Verification items for this drawing (mm, ordinates from the low corner). Give positions to 0.01 mm unless a question says otherwise; leave off trailing zeros. Write each loop counter-clockwise with the first axis right and the second up, starting at its lowest first coordinate (ties: lowest second). Pieces come first, ordered by that corner, then holes. Notation, with made-up numbers: M 71.25,-3.5 L 79.25,-3.5 A21 cw 79.25,30.5 Z; hole C -21,-19 d11. An arc over 180 degrees is marked long. Use one line per item in the form item = value. Start each with the question number.
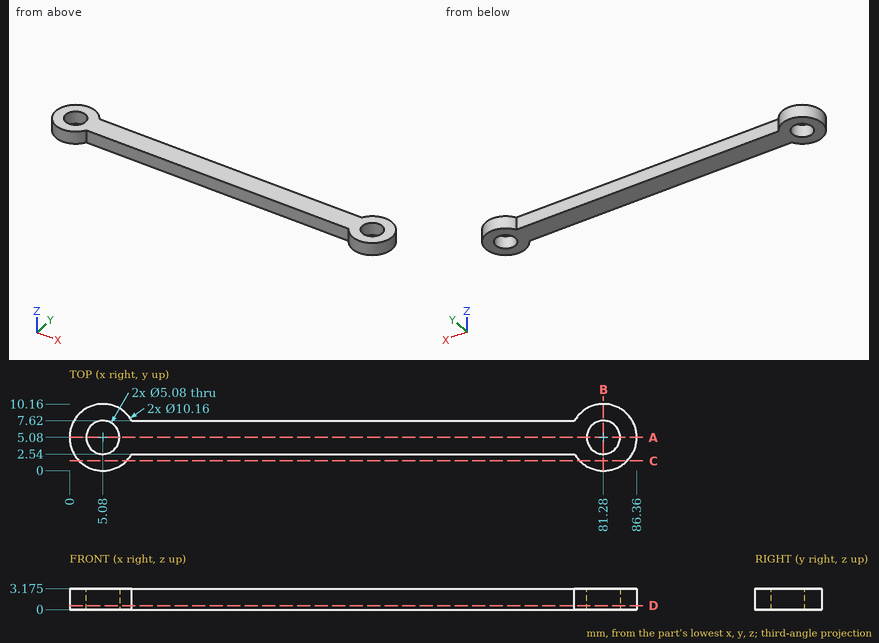
(1) Sectioned sample at C-C, the plane y = 1.5. Record the boundary of the cut face in (x, z) (3 decimals), plus the area to 3 significant figures.
(2) Sectioned sample at B-B, the plane x = 81.28. Record the boundary of the cut face in (y, z) (3 decimals).
(3) Thickness scan on probe 1 along X at (y, z) = (5, 0.7); probe 2 along X at (y, z) = (4.25, 2.3); probe 3 along Y at (x, z) = (81.28, 1.2). Record the ranges inside material, lowest first. Write a range as [from, to].
(4) Sectioned sample at A-A, the plane y = 5.08. Record the boundary of the cut face in (x, z) (3 decimals).
(5) Sectioned sample at D-D, the plane z = 0.6. Record the boundary of the cut face in (x, y).
(6) Depth check by flat-ended pin: pin 1 (1 mm diameter, centred on y = 2, z = 0.5, fed in from -X); pin 2 (1.5 mm diameter, centred on x = 58.5, z = 1.5, fed in from +Y). Enter the tip coordinate at first touch or a pass-through.
Numbers:
q1.outline = M 1.476,0 L 8.684,0 L 8.684,3.175 L 1.476,3.175 Z; M 77.676,0 L 84.884,0 L 84.884,3.175 L 77.676,3.175 Z
q1.area = 45.8 mm2
q2.outline = M 0,0 L 2.54,0 L 2.54,3.175 L 0,3.175 Z; M 7.62,0 L 10.16,0 L 10.16,3.175 L 7.62,3.175 Z
q3.probe_1 = [0, 2.54], [7.62, 78.74], [83.82, 86.36]
q3.probe_2 = [0.07, 2.68], [7.48, 78.88], [83.68, 86.29]
q3.probe_3 = [0, 2.54], [7.62, 10.16]
q4.outline = M 0,0 L 2.54,0 L 2.54,3.175 L 0,3.175 Z; M 7.62,0 L 78.74,0 L 78.74,3.175 L 7.62,3.175 Z; M 83.82,0 L 86.36,0 L 86.36,3.175 L 83.82,3.175 Z
q5.outline = M 9.48,2.54 L 76.88,2.54 A5.08 ccw long 76.88,7.62 L 9.48,7.62 A5.08 ccw long Z; hole C 5.08,5.08 d5.08; hole C 81.28,5.08 d5.08
q6.pin_1 = 0.7
q6.pin_2 = 7.62
